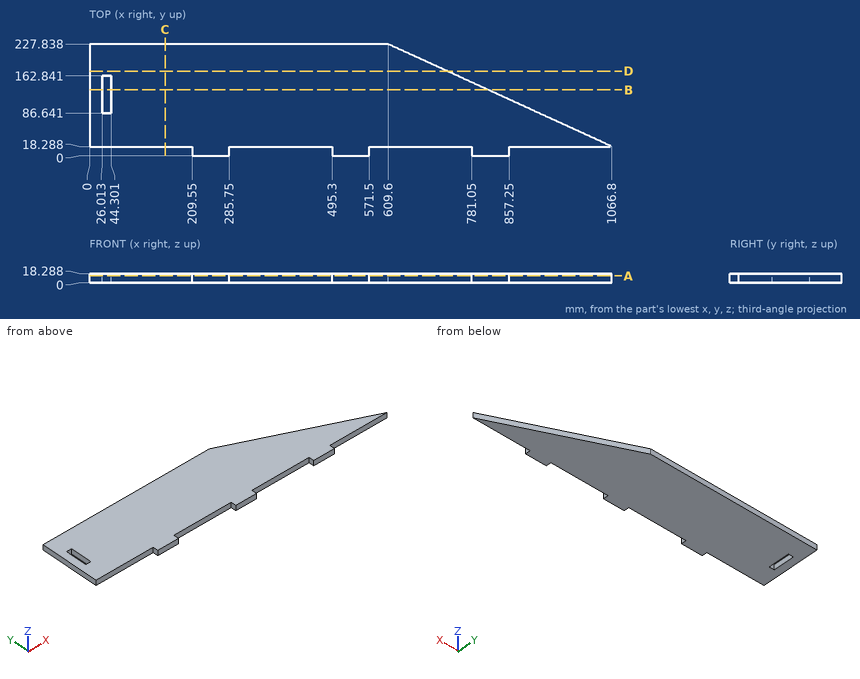
Here's the drawing with two shaded views (mm, measured from the low corner). I have some questions. Give positions to 0.01 mm unless a question says otherwise; leave off trailing zeros. Loops run counter-clockwise (first coordinate to the right, second up) from the corner with the lowest first, then second, coordinate; pieces in that order, holes last. Notation, with made-up numbers: (88, -31.5) - (108, -31.5) arc R23 ccw to (108, -13.5) - close; hole circle Ø2 at (76, -23.5). An arc over 180 degrees is marked (long way). Answer in a Markdown table with one row per item. Add a question column.
Q1. If we section it at B-B (y = 134): List the corners of the cut face in (x, z) for me.
Q2. Please list where these lines run through material, in increasing order: L1, parallel to X at y = 10.5, z = 11; L2, parallel to Y at x = 369.5, z = 11; L3, parallel to X at y = 122, z = 13 (1 decimal). Write a range as from..to.
Q3. For pin 1 (5.5 mm diameter, centred on x = 131, z = 13, fed in from -Y); pin 2 (5.5 mm diameter, centred on y = 117.5, z = 10, fed in from +X) (1 decimal); pin 3 (5 mm diameter, centred on y = 49.5, z = 8, fed in from +X) (1 decimal), each with a flat end and sliding along its axis, tell me the tip position at first contact or that it passes through.
Q4. If we section it at D-D (y = 172.5): List the corners of the cut face in (x, z) for me.
Q5. If we section it at A-A (z = 13.5): List the corners of the cut face in (x, y) for me, plus the area to 3 significant figures.
Q6. If we section it at C-C (x = 154.5): List the corners of the cut face in (y, z) for me.
The answers:
| question | item | result |
|---|---|---|
| 1 | outline | (0, 0) - (26.01, 0) - (26.01, 18.29) - (0, 18.29) - close; (44.3, 0) - (814.34, 0) - (814.34, 18.29) - (44.3, 18.29) - close |
| 2 | L1 | x = 209.55..285.75, 495.3..571.5, 781.05..857.25 |
| 2 | L2 | y = 18.29..227.84 |
| 2 | L3 | x = 0..26, 44.3..840.5 |
| 3 | pin 1 | stops at y = 18.29 |
| 3 | pin 2 | stops at x = 856.3 |
| 3 | pin 3 | stops at x = 1004.2 |
| 4 | outline | (0, 0) - (730.34, 0) - (730.34, 18.29) - (0, 18.29) - close |
| 5 | outline | (0, 18.29) - (209.55, 18.29) - (209.55, 0) - (285.75, 0) - (285.75, 18.29) - (495.3, 18.29) - (495.3, 0) - (571.5, 0) - (571.5, 18.29) - (781.05, 18.29) - (781.05, 0) - (857.25, 0) - (857.25, 18.29) - (1066.8, 18.29) - (609.6, 227.84) - (0, 227.84) - close; hole (26.01, 86.64) - (44.3, 86.64) - (44.3, 162.84) - (26.01, 162.84) - close |
| 5 | area | 178,000 mm^2 |
| 6 | outline | (18.29, 0) - (227.84, 0) - (227.84, 18.29) - (18.29, 18.29) - close |
